from build123d import *

# Parameters (mm, degrees)
SKETCH1_W           = 374.65
SKETCH1_H           = 263.525
SKETCH1_W_2         = 326.91662515
SKETCH1_H_2         = 223.901
BOSS_EXTRUDE1_DEPTH = 7.5
SKETCH1_2_W         = 326.91662515
SKETCH1_2_H         = 223.901
BOSS_EXTRUDE2_DEPTH = 7.1
FILLET1_R           = 7.62
FILLET2_R           = 7.62


with BuildPart() as part:
    # Sketch1 → Boss-Extrude1 (new body)
    with BuildSketch(Plane(origin=(0, 0, 0), x_dir=(1, 0, 0), z_dir=(0, 1, 0))):
        Rectangle(SKETCH1_W, SKETCH1_H)
        Rectangle(SKETCH1_W_2, SKETCH1_H_2, mode=Mode.SUBTRACT)
    extrude(amount=BOSS_EXTRUDE1_DEPTH)

    # Sketch1<2> → Boss-Extrude2 (add)
    with BuildSketch(Plane(origin=(0, 0, 0), x_dir=(1, 0, 0), z_dir=(0, 1, 0))):
        Rectangle(SKETCH1_2_W, SKETCH1_2_H)
    extrude(amount=BOSS_EXTRUDE2_DEPTH)

    # Fillet1
    # the kernel refuses this fillet: 7.62 mm, written as the material it takes off along each edge
    with BuildSketch(Plane(origin=(206.375, 0, -131.7625), x_dir=(0, 0, 1), z_dir=(-1, 0, 0))) as fillet1_piece_1:
        with BuildLine():
            CenterArc((FILLET1_R, FILLET1_R), FILLET1_R, 180, 90)
            Line((0, FILLET1_R), (0, 0))
            Line((0, 0), (FILLET1_R, 0))
        make_face()
    extrude(amount=412.75, mode=Mode.SUBTRACT)

    # Fillet2
    # the kernel refuses this fillet: 7.62 mm, written as the material it takes off along each edge
    with BuildSketch(Plane(origin=(-187.325, 0, -143.190137649), x_dir=(0, 1, 0), z_dir=(0, 0, 1)), Plane(origin=(187.325, 0, 150.810137649), x_dir=(0, 1, 0), z_dir=(0, 0, -1))) as fillet2_piece_1:
        with BuildLine():
            CenterArc((7.62, -7.61905506), FILLET2_R, 90.902333039, 89.097666961)
            Line((0, -7.61905506), (-0.1524, -7.61905506))
            Line((-0.1524, -7.61905506), (-0.1524, 0))
            Line((-0.1524, 0), (0, 0.1524))
            ThreePointArc((0, 0.1524), (3.75, 0.1524), (7.4976, 0.152381101))
            Line((7.4976, 0.152381101), (7.5, 0))
        make_face()
    extrude(amount=294.000275298, mode=Mode.SUBTRACT)
    with BuildSketch(Plane(origin=(-206.372637649, 0, 131.7625), x_dir=(0, 1, 0), z_dir=(1, 0, 0))) as fillet2_piece_2:
        with BuildLine():
            CenterArc((7.62, -7.61905506), FILLET2_R, 90.902333039, 89.097666961)
            Line((0, -7.61905506), (-0.1524, -7.61905506))
            Line((-0.1524, -7.61905506), (-0.1524, 0))
            Line((-0.1524, 0), (0, 0.1524))
            ThreePointArc((0, 0.1524), (3.75, 0.1524), (7.4976, 0.152381101))
            Line((7.4976, 0.152381101), (7.5, 0))
        make_face()
    extrude(amount=412.745275298, mode=Mode.SUBTRACT)


solid = part.part
For this review, take the finished solid that the model builds, in its own axes (mm). Give positions to 0.01 mm unless a question says otherwise; leave off trailing zeros. Loops run counter-clockwise (first coordinate to the right, second up) from the corner with the lowest first, then second, coordinate; pieces in that order, holes last. Notation, with made-up numbers: M 4.5,67 L 54.5,67 A13 cw 54.5,83 Z; hole C 81.25,36.25 d7. An arc over 180 degrees is marked long. Answer as a JSON object with one key per item and string values. Group by question number.
Q1. Add section B-B on x = 33.5. Give the boundary of the cut face in (y, z).
Q2. For probe 1 along Z at (x, y) = (-69.5, 7.25); probe 2 along Y at (x, z) = (73, 106.5); probe 3 along X at (y, z) = (6.75, -55), list the stretches that pass through material, from the lowest coordinate up. Write a range as [from, to].
Q3. Mouldability with a two-part tool opening along X and no side actions: class faces 1 (the cylindrical face through (-2.6, 2.2, 129.5)), 2 (the cylindrical face through (185.11, 2.25, 1.85)), 3 (the flat face through (-2, 7.1, -2)) as +X half, -X half, draft (parallel to the pull), parting line (faces both ways), or undercut.
Q4. Add section C-C on y = 2.25. Give the boundary of the cut face in (x, z).
Q5. Add section A-A on z = 101.5. Give the boundary of the cut face in (x, y) (3 decimals).
Q6. Insertion check: P1, Ø5, axis at x = 90, z = -23.5, coming from the +Y side; P2, Ø1.5, axis at x = 4.5, y = 3.5, coming from the +Z side; P3, Ø1, axis at x = 66.5, y = 3.5, coming from the -Z side. Each pin has a flat end and moves straight along its axis. Give the tip position at first contact, or say it passes through.
Checked values:
{
 "1": {"outline": "M 0,-124.14 A7.62 ccw 7.5,-131.76 L 7.5,-111.95 L 7.1,-111.95 L 7.1,111.95 L 7.5,111.95 L 7.5,131.76 A7.62 ccw 0,124.14 Z"},
 "2": {"probe 1": "[-131.75, -111.95], [111.95, 131.75]", "probe 2": "[0, 7.1]", "probe 3": "[-187.28, 187.28]"},
 "3": {"face 1": "draft", "face 2": "+X half", "face 3": "undercut"},
 "4": {"outline": "M -185.11,-129.55 L 185.11,-129.55 L 185.11,129.55 L -185.11,129.55 Z"},
 "5": {"outline": "M -187.325,7.5 A7.62 ccw -179.706,0 L 179.706,0 A7.62 ccw 187.325,7.5 L 163.458,7.5 L 163.458,7.1 L -163.458,7.1 L -163.458,7.5 Z"},
 "6": {"P1": "y = 7.1", "P2": "z = 130.98", "P3": "z = -130.85"}
}
